from build123d import *

# Parameters (mm, degrees)
SKETCH1_R           = 1.5
BOSS_EXTRUDE2_DEPTH = 10
SKETCH1_8_R         = 4
SKETCH1_8_R_2       = 1.5
BOSS_EXTRUDE4_DEPTH = 2
BOSS_EXTRUDE5_START = 2
SKETCH2_R           = 1.5
BOSS_EXTRUDE5_DEPTH = 2
CUT_EXTRUDE2_DEPTH  = 1.5
CHAMFER1_SIZE       = 2


with BuildPart() as part:
    # Sketch1 → Boss-Extrude2 (new body)
    with BuildSketch(Plane.XY):
        Circle(SKETCH1_R)
    extrude(amount=BOSS_EXTRUDE2_DEPTH)



with BuildPart() as body_2:
    # Sketch1<8> → Boss-Extrude4 (new body)
    with BuildSketch(Plane.XY):
        Circle(SKETCH1_8_R)
        Circle(SKETCH1_8_R_2, mode=Mode.SUBTRACT)
    extrude(amount=-BOSS_EXTRUDE4_DEPTH)


with BuildPart() as part_1:
    add(part.part)

    add(body_2.part)  # Boss-Extrude5 merges body 2
    # Sketch2 → Boss-Extrude5 (add)
    with BuildSketch(Plane(origin=(0, 0, 0), x_dir=(-1, 0, 0), z_dir=(0, 0, -1)).offset(BOSS_EXTRUDE5_START)):
        with Locations(Location((0, 0, 0), (0, 0, 180))):
            Circle(SKETCH2_R)
    extrude(amount=-BOSS_EXTRUDE5_DEPTH)

    # Sketch3 → Cut-Extrude2 (cut)
    with BuildSketch(Plane(origin=(0, 0, -2), x_dir=(-1, 0, 0), z_dir=(0, 0, -1))):
        Polygon((0, 1.947036768), (-1.686183303, 0.973518384), (-1.686183303, -0.973518384), (0, -1.947036768), (1.686183303, -0.973518384), (1.686183303, 0.973518384), align=None)
    extrude(amount=-CUT_EXTRUDE2_DEPTH, mode=Mode.SUBTRACT)

    # Chamfer1
    chamfer1_edges = [part_1.edges().sort_by_distance(p)[0] for p in [
        (-4, 0, -2),
    ]]
    chamfer(chamfer1_edges, length=CHAMFER1_SIZE - 0.0001)  # a hair under: the kernel refuses the full size


solid = part_1.part
Geometry: final body of the model. Coordinates: model frame, mm. A direction names the side the tool comes from. Round coordinates to 2 decimals unless told otherwise and drop trailing zeros. Order: outer loops, then holes, each group sorted by start corner. A loop starts at its lowest first (then second) coordinate and runs counter-clockwise, first axis right, second up.
Q1. Section B-B, the plane z = -0.75. Output: boundary loops of the cut face in (x, y).
Result sheet:
outline: circle Ø6.5 at (0, 0); hole (-1.69, -0.97) - (0, -1.95) - (1.69, -0.97) - (1.69, 0.97) - (0, 1.95) - (-1.69, 0.97) - close
Q2. Mould query, pull axis Y, two halves, no side actions, for faces 1 (the face through (0, 0, 10)), 2 (the face through (-0.83, -1.47, -1.26)), 3 (the face through (-1.5, 0.07, 4.93)). Classes: released by +Y, released by -Y, zero draft, split by the parting line, or undercut.
Result sheet:
face 1: zero draft
face 2: undercut
face 3: split by the parting line
Q3. Section C-C, the plane z = 2.5. Output: boundary loops of the cut face in (x, y), and give its area (3 significant figures).
Result sheet:
outline: circle Ø3 at (0, 0)
area: 7.07 mm2
Q4. Pin query (flat end, axial travel): pin 1 (1.5 mm diameter, centred on x = -2.5, y = -2.5, fed in from +Z); pin 2 (1.6 mm diameter, centred on y = 0, z = -1, fed in from +X); pin 3 (0.8 mm diameter, centred on y = 0, z = -1, fed in from -X). Return the tip coordinate at first contact, or that it passes through.
Result sheet:
pin 1: stops at z = 0
pin 2: stops at x = 3.8
pin 3: stops at x = -3.4
Q5. Material intervals for probe 1 along Z at (x, y) = (-0.5, 0); probe 2 along Y at (x, z) = (-1, -1.5); probe 3 along Z at (x, y) = (-2.25, 3), sorted ascending.
Result sheet:
probe 1: z = -0.5 to 10
probe 2: y = -2.29 to -1.37, 1.37 to 2.29
probe 3: z = -0.25 to 0
Q6. Access query for faces 4 (the face through (2, 0, 0)), 5 (the face through (0.83, 1.47, -1.26)). Directions: +Z, -Z, +X, -X, +Y, -Y. A direction counts if a zero-diameter tool reaches every point of the face in a straight line with its end or side. Return the directions, or none.
Result sheet:
face 4: +Z
face 5: -Z
